Build history of the part. All positions in model axes, mm. Face numbers are marked on the shaded views. A direction names the side the tool comes from. Coordinates: 2 decimals unless noted, no trailing zeros. Loops run counter-clockwise (first coordinate to the right, second up) from the corner with the lowest first, then second, coordinate; pieces in that order, holes last.
(1) Slice it at A-A (x = -80). Give the cut face in (y, z).
(2) Wall check: L1, parallel to X at y = 25, z = 10; L2, parallel to Y at x = -68.5, z = 30; L3, parallel to Y at x = -163, z = 5. Give the ranges that are in metal, low to high.
(3) Flat gauge pins, fed straight in: P1, Ø2, axis at x = -44.71, y = 28.21, coming from the -Z side; P2, Ø4, axis at y = 39.5, z = 26, coming from the -X side; P3, Ø15.5, axis at x = -109.5, z = 14, coming from the +Y side; P4, Ø3, axis at x = -141.73, y = 25, coming from the -Z side. Where does each tip first touch, or does it go through?
(4) Slice it at B-B (z = 17). Give the cut face in (x, y).
(5) Tool access for the marked faces 1, 2 and 3: list every direction of +Z, -Z, +X, -X, +Y, -Y with a clear straight run to the whole face (end or side of a thin tool).
from build123d import *

# Parameters (mm, degrees)
SKETCH_1_R           = 1.25
EXTRUDE_1_DEPTH      = 29
EXTRUDE_2_DEPTH      = 3
EXTRUDE_2_DEPTH_BACK = 32
CHAMFER_1_SIZE       = 2


with BuildPart() as part:
    # 草图1 → 凸台-拉伸1 (new body)
    with BuildSketch(Plane.XY):
        with BuildLine():
            Line((-71.271215686, 33), (-163.728784314, 33))
            ThreePointArc((-163.728784314, 33), (-187.426920576, 35.752824596), (-209.86299145, 43.864694254))
            ThreePointArc((-209.86299145, 43.864694254), (-211.371961919, 43.977504611), (-212.528051157, 43.001197422))
            Line((-212.528051157, 43.001197422), (-213, 42.09809972))
            ThreePointArc((-213, 42.09809972), (-202.192009237, 35.020119991), (-192.973824319, 25.968295413))
            ThreePointArc((-192.973824319, 25.968295413), (-190.288164523, 24.71302347), (-187.602714776, 25.968744715))
            ThreePointArc((-187.602714776, 25.968744715), (-184.680917301, 28.037551849), (-181.118358374, 28.391158027))
            ThreePointArc((-181.118358374, 28.391158027), (-172.451349972, 27.34834419), (-163.728784314, 27))
            Line((-163.728784314, 27), (-150.96187697, 27))
            ThreePointArc((-150.96187697, 27), (-147.37951276, 26.013872851), (-144.806481866, 23.333333333))
            ThreePointArc((-144.806481866, 23.333333333), (-141.728784314, 21.5), (-138.651086762, 23.333333333))
            ThreePointArc((-138.651086762, 23.333333333), (-136.078055868, 26.013872851), (-132.495691658, 27))
            Line((-132.495691658, 27), (-102.504308342, 27))
            ThreePointArc((-102.504308342, 27), (-98.921944132, 26.013872851), (-96.348913238, 23.333333333))
            ThreePointArc((-96.348913238, 23.333333333), (-93.271215686, 21.5), (-90.193518134, 23.333333333))
            ThreePointArc((-90.193518134, 23.333333333), (-87.62048724, 26.013872851), (-84.03812303, 27))
            Line((-84.03812303, 27), (-71.271215686, 27))
            ThreePointArc((-71.271215686, 27), (-62.548650028, 27.34834419), (-53.881641626, 28.391158027))
            ThreePointArc((-53.881641626, 28.391158027), (-50.319082699, 28.037551849), (-47.397285224, 25.968744715))
            ThreePointArc((-47.397285224, 25.968744715), (-44.711835477, 24.71302347), (-42.026175681, 25.968295413))
            ThreePointArc((-42.026175681, 25.968295413), (-32.807990763, 35.020119991), (-22, 42.09809972))
            Line((-22, 42.09809972), (-22.471948843, 43.001197422))
            ThreePointArc((-22.471948843, 43.001197422), (-23.628038081, 43.977504611), (-25.13700855, 43.864694254))
            ThreePointArc((-25.13700855, 43.864694254), (-47.573079424, 35.752824596), (-71.271215686, 33))
        make_face()
        with Locations(Location((-44.711542697, 28.213023457, 0), (0, 0, 180))):
            Circle(SKETCH_1_R, mode=Mode.SUBTRACT)
        with Locations(Location((-93.271215686, 25, 0), (0, 0, 180))):
            Circle(SKETCH_1_R, mode=Mode.SUBTRACT)
        with Locations(Location((-141.728784314, 25, 0), (0, 0, 180))):
            Circle(SKETCH_1_R, mode=Mode.SUBTRACT)
        with Locations(Location((-190.288457303, 28.213023457, 0), (0, 0, 180))):
            Circle(SKETCH_1_R, mode=Mode.SUBTRACT)
    extrude(amount=EXTRUDE_1_DEPTH)

    # 草图2 → 凸台-拉伸2 (add, two sides: drawn at the far end of the back side and taken through both)
    with BuildSketch(Plane(origin=(0, 0, 0), x_dir=(-1, 0, 0), z_dir=(0, 0, -1)).offset(-EXTRUDE_2_DEPTH_BACK)):
        with BuildLine():
            Line((163.728784314, 30), (71.271215686, 30))
            ThreePointArc((71.271215686, 30), (45.903831548, 33.068787794), (22, 42.09809972))
            Line((22, 42.09809972), (22.471948843, 43.001197422))
            ThreePointArc((22.471948843, 43.001197422), (23.628038081, 43.977504611), (25.13700855, 43.864694254))
            ThreePointArc((25.13700855, 43.864694254), (47.573079424, 35.752824596), (71.271215686, 33))
            Line((71.271215686, 33), (163.728784314, 33))
            ThreePointArc((163.728784314, 33), (187.426920576, 35.752824596), (209.86299145, 43.864694254))
            ThreePointArc((209.86299145, 43.864694254), (211.371961919, 43.977504611), (212.528051157, 43.001197422))
            Line((212.528051157, 43.001197422), (213, 42.09809972))
            ThreePointArc((213, 42.09809972), (189.096168452, 33.068787794), (163.728784314, 30))
        make_face()
    extrude(amount=EXTRUDE_2_DEPTH + EXTRUDE_2_DEPTH_BACK)

    # 倒角1
    chamfer_1_edges = [part.edges().sort_by_distance(p)[0] for p in [
        (-22.235974422, 42.549648571, 32),
        (-23.628038081, 43.977504611, 32),
        (-47.573079424, 35.752824596, 32),
        (-117.5, 33, 32),
        (-187.426920576, 35.752824596, 32),
        (-211.371961919, 43.977504611, 32),
        (-212.764025578, 42.549648571, 32),
        (-212.764025578, 42.549648571, -3),
        (-211.371961919, 43.977504611, -3),
        (-187.426920576, 35.752824596, -3),
        (-117.5, 33, -3),
        (-47.573079424, 35.752824596, -3),
        (-23.628038081, 43.977504611, -3),
        (-22.235974422, 42.549648571, -3),
    ]]
    chamfer(chamfer_1_edges, length=CHAMFER_1_SIZE - 0.0001)  # a hair under: the kernel refuses the full size


solid = part.part
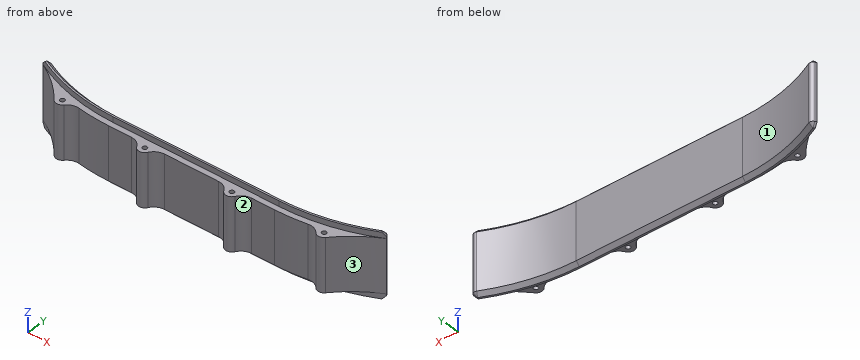
Response values:
1. outline: (27, 0) - (30, 0) - (30, -3) - (31, -3) - (33, -1) - (33, 30) - (31, 32) - (30, 32) - (30, 29) - (27, 29) - close
2. L1: x = -191.68 to -188.9, -146.06 to -142.98, -140.48 to -137.39, -97.61 to -94.52, -92.02 to -88.94, -46.1 to -43.32
2. L2: y = 30.04 to 33.04
2. L3: y = 27 to 33
3. P1: passes through
3. P2: stops at x = -211.88
3. P3: stops at y = 33
3. P4: stops at z = 0
4. outline: (-213, 42.1) arc R65.86 cw to (-192.97, 25.97) arc R3.5 ccw to (-187.6, 25.97) arc R7 cw to (-181.12, 28.39) arc R109.38 ccw to (-163.73, 27) - (-150.96, 27) arc R7 cw to (-144.81, 23.33) arc R3.5 ccw to (-138.65, 23.33) arc R7 cw to (-132.5, 27) - (-102.5, 27) arc R7 cw to (-96.35, 23.33) arc R3.5 ccw to (-90.19, 23.33) arc R7 cw to (-84.04, 27) - (-71.27, 27) arc R109.38 ccw to (-53.88, 28.39) arc R7 cw to (-47.4, 25.97) arc R3.5 ccw to (-42.03, 25.97) arc R65.86 cw to (-22, 42.1) - (-22.47, 43) arc R2 ccw to (-25.14, 43.86) arc R103.38 cw to (-71.27, 33) - (-163.73, 33) arc R103.38 cw to (-209.86, 43.86) arc R2 ccw to (-212.53, 43) - close; hole circle Ø2.5 at (-190.29, 28.21); hole circle Ø2.5 at (-141.73, 25); hole circle Ø2.5 at (-93.27, 25); hole circle Ø2.5 at (-44.71, 28.21)
5. face 1: +Z, -Z, +Y
5. face 2: +Z, -Z, -Y
5. face 3: +Z, -Z, +X, -Y
